Geometry: final body of the model. Coordinates: model frame, mm. A direction names the side the tool comes from. Coordinates: 2 decimals unless noted, no trailing zeros. Order: outer loops, then holes, each group sorted by start corner. A loop starts at its lowest first (then second) coordinate and runs counter-clockwise, first axis right, second up. Notation, with made-up numbers: (46, 1) -> (68, 1) arc R30 ccw to (68, 24) -> close; hole circle Ø6 at (-38.5, 57). An arc over 180 degrees is marked (long way). Use CSV: the item, a comma, the result in double quotes. Start each with the question number.
Autodesk Inventor part; units mm, degrees
ref_plane "Work Plane1" through (-50, 55, 0) normal (-1, 0, 0) x (0, -1, 0)
ref_plane "Work Plane2" through (-62.5, 34.7882, 0) normal (0, 1, 0) x (1, 0, 0)
ref_plane "Work Plane7" through (22.6604, 3.5721, 0) normal (-0.766, 0.6428, 0) x (0, 0, 1)
sketch "Sketch1" plane through (0, 0, 0) normal (0, 1, 0) x (-1, 0, 0)
  circle A0 centre (0, 0) radius 50
  dimension "d0" = 100
extrude "Extrusion1" add sketch "Sketch1" along normal blind 60
sketch "Sketch2" plane through (0, 60, 0) normal (0, 1, 0) x (1, 0, 0)
  circle A0 centre (0, 0) radius 50
  circle A1 centre (0, 50) radius 7.5
  circle A2 centre (43.3013, 25) radius 7.5
  circle A3 centre (43.3013, -25) radius 7.5
  circle A4 centre (0, -50) radius 7.5
  circle A5 centre (-43.3013, -25) radius 7.5
  circle A6 centre (-43.3013, 25) radius 7.5
  dimension "d3" = 15
  dimension "d6" = 360
fillet "Fillet1" radius 5 1 edges at (50, 60, 0)
extrude "Extrusion2" cut sketch "Sketch2" against normal blind 5 contours A2 A0 | A0 A2 | A3 A0 | A0 A3 | A1 A0 | A0 A1 | A4 A0 | A0 A4 | A6 A0 | A0 A6 | A5 A0 | A0 A5
ref_plane "Work Plane1" through (-50, 55, 0) normal (-1, 0, 0) x (0, -1, 0)
sketch "Sketch4" plane through (-50, 55, 0) normal (-1, 0, 0) x (0, -1, 0)
  line L0 (27.2118, -30) -> (42.2118, -30)
  line L1 (42.2118, -30) -> (42.2118, 30)
  line L2 (42.2118, 30) -> (27.2118, 30)
  line L3 (27.2118, 30) -> (27.2118, -30)
  point P0 (55, 0)
  dimension "d14" = 60
  dimension "d15" = 15
extrude "Extrusion4" add sketch "Sketch4" along normal mid plane 70
sketch "Sketch5" plane through (-50, 55, 0) normal (-1, 0, 0) x (0, -1, 0)
  line L0 (27.2118, 30) -> (27.2118, -30)
  line L1 (27.2118, 14) -> (20.2118, 14)
  line L2 (20.2118, 14) -> (20.2118, -14)
  line L3 (20.2118, -14) -> (27.2118, -14)
  line L4 (27.2118, -14) -> (27.2118, 14)
  point P0 (55, 0)
  dimension "d18" = 7
  dimension "d19" = 28
extrude "Extrusion5" add sketch "Sketch5" along normal mid plane 25
fillet "Fillet2" radius 8 2 edges at (-85, 20.2882, -30) (-85, 20.2882, 30)
sketch "Sketch6" plane through (-62.5, 27.7882, 14) normal (0, 1, 0) x (1, 0, 0)
  point P0 (62.5, 14)
ref_plane "Work Plane2" through (-62.5, 34.7882, 0) normal (0, 1, 0) x (1, 0, 0)
sketch "Sketch7" plane through (-62.5, 34.7882, 0) normal (0, 1, 0) x (1, 0, 0)
  line L0 (6.0723, 20.1953) -> (-8.4303, 6.4231)
  line L1 (-8.4303, 6.4231) -> (-11.1847, 9.3236)
  line L2 (-11.1847, 9.3236) -> (3.3179, 23.0958)
  line L3 (3.3179, 23.0958) -> (6.0723, 20.1953)
  line L4 (11.5119, 0) -> (-21.1929, 0)
  line L5 (6.0723, -20.1953) -> (-8.4303, -6.4231)
  line L6 (-8.4303, -6.4231) -> (-11.1847, -9.3236)
  line L7 (-11.1847, -9.3236) -> (3.3179, -23.0958)
  line L8 (3.3179, -23.0958) -> (6.0723, -20.1953)
  point P0 (62.5, 0)
  dimension "d23" = 20
  dimension "d24" = 4
extrude "Extrusion6" cut sketch "Sketch7" against normal blind 50
fillet "Fillet3" radius 4 2 edges at (-62.5, 31.2882, -14) (-62.5, 31.2882, 14)
sketch "Sketch11" plane through (0, 0, 0) normal (0, 0, 1) x (1, 0, 0)
  line L0 (-15, 10) -> (15, 10)
  line L1 (15, 10) -> (15, 30)
  line L2 (15, 30) -> (-15, 30)
  line L3 (-15, 30) -> (-15, 10)
  point P0 (0, 0)
  dimension "d29" = 30
  dimension "d30" = 20
extrude "Extrusion7" cut sketch "Sketch11" along normal mid plane 100
sketch "Sketch12" plane through (0, 0, 0) normal (0, 0, 1) x (1, 0, 0)
  line L0 (-15, 10) -> (15, 10)
  line L1 (15, 10) -> (15, 30)
  line L2 (15, 30) -> (-15, 30)
  line L3 (-15, 30) -> (-15, 10)
  point P0 (0, 0)
  dimension "d33" = 30
  dimension "d34" = 20
extrude "Extrusion8" add sketch "Sketch12" along normal mid plane 40
ref_plane "Work Plane7" through (22.6604, 3.5721, 0) normal (-0.766, 0.6428, 0) x (0, 0, 1)
ref_plane "Work Plane6" through (15, 10, 0) normal (-0.766, 0.6428, 0) x (0, 0, 1)
ref_plane "Work Plane8" through (20, 0, 0) normal (1, 0, 0) x (0, 1, 0)
sketch "Sketch18" plane through (20, 0, 0) normal (1, 0, 0) x (0, 1, 0)
  line L0 (10, 25) -> (35, 25)
  line L1 (35, 25) -> (35, -25)
  line L2 (35, -25) -> (10, -25)
  line L3 (10, -25) -> (10, 25)
  dimension "d52" = 25
  dimension "d53" = 50
extrude "Extrusion11" cut sketch "Sketch18" along normal blind 30
properties part number "redondogas"
(1) Section A-A (y = 16). Return loops of the section in (x, z).
(2) Line query: line 1 (Y direction, x = 39.5, z = 15); line 2 (Z direction, x = 9.5, y = 12); line 3 (X direction, y = 10.5, z = 27). Output: solid intervals per line, ascending. Write a range as from..to.
(3) Mould query, pull axis X, two halves, no side actions, for faces 4 (the face through (-61.359, 31.337, 12.797)), 5 (the face through (-36.729, 57.535, 21.387)), 6 (the face through (31, 23, -25)). Classes: pulls with the +X half, pulls with the -X half, needs draft (parallel to the pull), parting line crosses it, or undercut.
(4) Section B-B (x = -52). Return loops of the section in (y, z).
(5) Section D-D (y = 39). Return loops of the section in (x, z).
(6) First-contact query: pin 1 (7.5 mm diameter, centred on y = 16.5, z = 1.5, fed in from +X); pin 2 (7 mm diameter, centred on x = 34, y = 19.5, fed in from -Z); pin 3 (2 mm diameter, centred on y = 51.5, z = 37, fed in from -X); pin 4 (24 mm diameter, centred on x = -2, z = -35.5, fed in from -Y). Flat tips, straight axial feed; report the tip coordinate or a pass-through.
(7) Section C-C (z = 0). Return loops of the section in (x, y).
(8) Access query for faces 1 (the face through (-15, 20, 34)), 2 (the face through (-61.359, 31.239, -12.797)), 3 (the face through (-72.288, 20.393, -7.853)). Directions: +Z, -Z, +X, -X, +Y, -Y. A direction counts if a zero-diameter tool reaches every point of the face in a straight line with its end or side. Return the directions, or none.
Check sheet entries:
1,outline,"(-85, -22) arc R8 ccw to (-77, -30) -> (-40, -30) arc R50 ccw to (-15, -47.7) -> (-15, -20) -> (15, -20) -> (15, -47.7) arc R50 ccw to (43.3, -25) -> (20, -25) -> (20, 25) -> (43.3, 25) arc R50 ccw to (15, 47.7) -> (15, 20) -> (-15, 20) -> (-15, 47.7) arc R50 ccw to (-40, 30) -> (-77, 30) arc R8 ccw to (-85, 22) -> close; hole (-73.68, -9.32) -> (-59.18, -23.1) -> (-56.43, -20.2) -> (-70.93, -6.42) -> close; hole (-73.68, 9.32) -> (-70.93, 6.42) -> (-56.43, 20.2) -> (-59.18, 23.1) -> close"
2,line 1,"y = 0..10, 35..60"
2,line 2,"z = -20..20"
2,line 3,"x = -42.08..-15, 15..42.08"
3,face 4,"pulls with the -X half"
3,face 5,"undercut"
3,face 6,"needs draft"
4,outline,"(12.79, -30) -> (27.79, -30) -> (27.79, -14) -> (34.79, -14) -> (34.79, 14) -> (27.79, 14) -> (27.79, 30) -> (12.79, 30) -> close"
5,outline,"circle Ø100 at (0, 0)"
6,pin 1,"stops at x = 20"
6,pin 2,"stops at z = -39.62"
6,pin 3,"stops at x = -34.7"
6,pin 4,"stops at y = 0"
7,outline,"(-85, 12.79) -> (-50, 12.79) -> (-50, 0) -> (50, 0) -> (50, 10) -> (20, 10) -> (20, 35) -> (50, 35) -> (50, 55) arc R5 ccw to (45, 60) -> (-45, 60) arc R5 ccw to (-50, 55) -> (-50, 34.79) -> (-62.5, 34.79) -> (-62.5, 27.79) -> (-85, 27.79) -> close"
8,face 1,"+Z"
8,face 2,"-Z, -X, +Y"
8,face 3,"+Y, -Y"
